Input: part model. Units: mm. Frame: model coordinates. Face numbers are marked on the shaded views. A direction names the side the tool comes from. Round coordinates to 2 decimals unless told otherwise and drop trailing zeros. Loops run counter-clockwise (first coordinate to the right, second up) from the corner with the lowest first, then second, coordinate; pieces in that order, holes last. Notation, with made-up numbers: (-9.75, -3.75) -> (10.25, -3.75) arc R13 ccw to (10.25, 14.25) -> close; hole circle Ø10 at (62, -25). An arc over 180 degrees is marked (long way). Answer as a JSON object with one key per item and string values. Group by question number.
Item 1: Section query D-D on y = 6. Return loops of the section in (x, z), and give its area (3 significant figures).
Item 2: Set-up query: the marked faces 4, 5, 6 and 7. Return all of +Z, -Z, +X, -X, +Y, -Y with unobstructed straight access to the full face (end or side cutting, diameter ignored); none if empty.
Item 3: Material intervals for line 1 (Z direction, x = 0, y = 3.7); line 2 (X direction, y = 11.75, z = 14.5); line 3 (X direction, y = 3.9, z = 10), sorted ascending. Write a range as [from, to].
Item 4: Section query A-A on z = 14. Return loops of the section in (x, y).
Item 5: Section query C-C on y = 10. Count the separate pieces of the cut face and the enclosed holes in it, and give its area (3 significant figures).
Item 6: Section query B-B on y = 4.5. Return loops of the section in (x, z), and give its area (3 significant figures).
Item 7: Draft query along Z for the marked faces 1, 2 and 3. Return one class per face: released by +Z, released by -Z, zero draft, split by the parting line, or undercut.
Item 8: Pin query (flat end, axial travel): pin 1 (2 mm diameter, centred on x = -3.5, y = 3, fed in from +Z); pin 2 (4 mm diameter, centred on x = -3, y = 4.5, fed in from +Z); pin 3 (1 mm diameter, centred on y = 7.5, z = 8, fed in from -X). Return the tip coordinate at first contact, or that it passes through.
from build123d import *

# Parameters (mm, degrees)
RESSALTO_EXTRUS_O1_DEPTH   = 20
INCLINA_O1_DEPTH           = 20
INCLINA_O1_START           = -6
INCLINA_O1_2_DEPTH         = 12
CORTE_EXTRUS_O1_DEPTH      = 25.372115214
CORTE_EXTRUS_O1_DEPTH_BACK = 25.372115214
M5_GEWINDEBOHRUNG1_D       = 4.2
M5_GEWINDEBOHRUNG1_DEPTH   = 5
M5_GEWINDEBOHRUNG1_TIP     = 1.2618073


with BuildPart() as part:
    # Esboço1 → Ressalto-extrusão1 (new body)
    with BuildSketch(Plane.XY):
        Polygon((-5, 0), (5, 0), (3.5, 13), (1.5, 13), (0.25, 8), (-0.25, 8), (-1.5, 13), (-3.5, 13), align=None)
    extrude(amount=RESSALTO_EXTRUS_O1_DEPTH)

    # Inclinação1: read off the stored shape, not the designer's step
    # Inclinação1 outline → Inclinação1 (cut)
    with BuildSketch(Plane.XY):
        Polygon((3.5, 13), (3.403800708, 13), (5, 0), align=None)
        Polygon((-5, 0), (-3.403800708, 13), (-3.5, 13), align=None)
    extrude(amount=INCLINA_O1_DEPTH, mode=Mode.SUBTRACT)

    # Inclina_o1 2 outline → Inclina_o1 2 (cut)
    with BuildSketch(Plane.YZ.offset(INCLINA_O1_START)):
        Polygon((13, 18.403800708), (13, 20), (0, 20), align=None)
        Polygon((13, 0), (13, 1.596199292), (0, 0), align=None)
    extrude(amount=INCLINA_O1_2_DEPTH, mode=Mode.SUBTRACT)

    # Esboço3 → Corte-extrusão1 (cut, two sides: drawn at the far end of the back side and taken through both)
    with BuildSketch(Plane(origin=(0, 0, 0), x_dir=(0, 0, -1), z_dir=(1, 0, 0)).offset(-CORTE_EXTRUS_O1_DEPTH_BACK)):
        Polygon((-17.5, 13), (-16.25, 8), (-15.75, 8), (-14.5, 13), align=None)
        Polygon((-13.5, 13), (-12.25, 8), (-11.75, 8), (-10.5, 13), align=None)
        Polygon((-9.5, 13), (-8.25, 8), (-7.75, 8), (-6.5, 13), align=None)
        Polygon((-5.5, 13), (-4.25, 8), (-3.75, 8), (-2.5, 13), align=None)
    extrude(amount=CORTE_EXTRUS_O1_DEPTH + CORTE_EXTRUS_O1_DEPTH_BACK, mode=Mode.SUBTRACT)

    # M5 Gewindebohrung1
    with Locations(Plane(origin=(0, 0, 10), x_dir=(-1, 0, 0), z_dir=(0, -1, 0))):
        with Locations((0, 0)):
            Hole(M5_GEWINDEBOHRUNG1_D / 2, depth=M5_GEWINDEBOHRUNG1_DEPTH)
            with Locations((0, 0, -(M5_GEWINDEBOHRUNG1_DEPTH + M5_GEWINDEBOHRUNG1_TIP / 2))):  # 118° drill point
                Cone(0, M5_GEWINDEBOHRUNG1_D / 2, M5_GEWINDEBOHRUNG1_TIP, mode=Mode.SUBTRACT)


solid = part.part
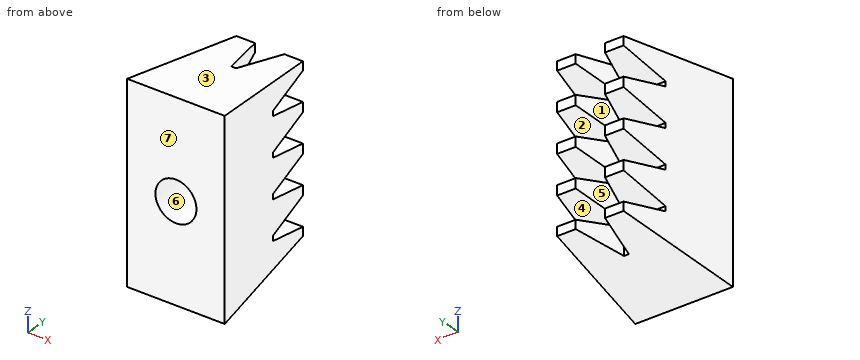
Solved:
{
 "1": {"outline": "(-4.26, 0.74) -> (4.26, 0.74) -> (4.26, 19.26) -> (-4.26, 19.26) -> close; hole circle Ø0.87 at (0, 10)", "area": "157 mm²"},
 "2": {"face 4": "+X, -X, +Y", "face 5": "+Z, -Z, +Y", "face 6": "-Y", "face 7": "+Z, -Z, +X, -X, -Y"},
 "3": {"line 1": "[0.45, 7.9], [12.1, 19.55]", "line 2": "[-3.56, -1.19], [1.19, 3.56]", "line 3": "[-4.52, -2.1], [2.1, 4.52]"},
 "4": {"outline": "(-5, 0) -> (5, 0) -> (3.4, 13) -> (1.5, 13) -> (0.25, 8) -> (-0.25, 8) -> (-1.5, 13) -> (-3.4, 13) -> close"},
 "5": {"separate pieces": "10", "enclosed holes": "0", "area": "69.8 mm²"},
 "6": {"outline": "(-4.45, 0.55) -> (4.45, 0.55) -> (4.45, 19.45) -> (-4.45, 19.45) -> close; hole circle Ø4.2 at (0, 10)", "area": "154 mm²"},
 "7": {"face 1": "zero draft", "face 2": "undercut", "face 3": "released by +Z"},
 "8": {"pin 1": "z = 19.75", "pin 2": "z = 19.69", "pin 3": "x = -4.14"}
}
